Work out the finished part from the listing and answer in its coordinate system (mm). A direction names the side the tool comes from. Coordinates: 2 decimals unless noted, no trailing zeros. Order: outer loops, then holes, each group sorted by start corner. A loop starts at its lowest first (then second) coordinate and runs counter-clockwise, first axis right, second up.
1. The part is cut by section C-C, the plane z = -28. Give the vertices of the cut face in (x, y), then the cut area to 3 significant figures.
2. A tool of negligible diameter and unlimited length cuts with its end or side. For faces 1 (the flat face through (-13.65, 0.02, -21.52)), 2 (the flat face through (-16.895, 0.022, -9.243)), 3 (the flat face through (-14.65, 0.02, -23.84)), 4 (the flat face through (13.61, 0.02, -21.51)), from which of +Z, -Z, +X, -X, +Y, -Y can it reach the whole face along a straight path? Write none if from no direction.
3. The part is cut by section A-A, the plane x = 0. Give the vertices of the cut face in (y, z), then the cut area to 3 significant figures.
4. The part is cut by section D-D, the plane x = -18. Give the vertices of the cut face in (y, z).
5. Find the intervals of material crossed by probe 1 along Z at (x, y) = (0, 0.9); probe 2 along Z at (x, y) = (-2, 1.2); probe 3 along X at (y, z) = (1.1, -21), in increasing order.
6. The part is cut by section B-B, the plane y = -0.05. Give the vertices of the cut face in (x, z), then the cut area to 3 significant figures.
7. Determine the mould class of faces 5 (the flat face through (0, 0, 0)), 6 (the flat face through (19.762, 0.022, -4.762)), 7 (the cylindrical face through (3.53, -0.022, -15.126)), 8 (the flat face through (16.938, 0.022, -9.254)) for opening direction X: +X half, -X half, draft (parallel to the pull), parting line (faces both ways), or undercut.
8. A flat-ended cylindrical pin translates along its axis: pin 1 Ø1 at (y, z) = (0.5, -14.5) entering from -X. Find the tip coordinate at first contact, or state that the pin passes through.
```python
from build123d import *

# Parameters (mm, degrees)
SKETCH1_R           = 7.65
BOSS_EXTRUDE1_DEPTH = 1.5875


with BuildPart() as part:
    # Sketch1 → Boss-Extrude1 (new, symmetric)
    with BuildSketch(Plane(origin=(0, 0, 0), x_dir=(1, 0, 0), z_dir=(0, 1, 0))):
        with BuildLine():
            Line((-18.450042271, 9.659258263), (-21.038232722, 0))
            Line((-21.038232722, 0), (21.038232722, 0))
            Line((21.038232722, 0), (18.450042271, 9.659258263))
            Line((18.450042271, 9.659258263), (15.383227773, 8.837507795))
            Line((15.383227773, 8.837507795), (12.0962259, 21.104765789))
            Line((12.0962259, 21.104765789), (15.163040398, 21.926516257))
            Line((15.163040398, 21.926516257), (14.150813355, 25.704199011))
            ThreePointArc((14.150813355, 25.704199011), (0, 36.5625), (-14.150813355, 25.704199011))
            Line((-14.150813355, 25.704199011), (-15.163040398, 21.926516257))
            Line((-15.163040398, 21.926516257), (-12.0962259, 21.104765789))
            Line((-12.0962259, 21.104765789), (-15.383227773, 8.837507795))
            Line((-15.383227773, 8.837507795), (-18.450042271, 9.659258263))
        make_face()
        with Locations((0, 21.9125)):
            Circle(SKETCH1_R, mode=Mode.SUBTRACT)
    extrude(amount=BOSS_EXTRUDE1_DEPTH, both=True)


solid = part.part
```
Geometry says:
1. outline: (-13.33, -1.59) - (-4.63, -1.59) - (-4.63, 1.59) - (-13.33, 1.59) - close; (4.63, -1.59) - (13.33, -1.59) - (13.33, 1.59) - (4.63, 1.59) - close
1. area: 55.2 mm2
2. face 1: -X, +Y, -Y
2. face 2: -Z, +Y, -Y
2. face 3: -Z, -X, +Y, -Y
2. face 4: +X, +Y, -Y
3. outline: (-1.59, -36.56) - (1.59, -36.56) - (1.59, -29.56) - (-1.59, -29.56) - close; (-1.59, -14.26) - (1.59, -14.26) - (1.59, 0) - (-1.59, 0) - close
3. area: 67.5 mm2
4. outline: (-1.59, -9.54) - (1.59, -9.54) - (1.59, 0) - (-1.59, 0) - close
5. probe 1: z = -36.56 to -29.56, -14.26 to 0
5. probe 2: z = -36.43 to -29.3, -14.53 to 0
5. probe 3: x = -12.12 to -7.6, 7.6 to 12.12
6. outline: (-21.04, 0) - (-18.45, -9.66) - (-15.38, -8.84) - (-12.1, -21.1) - (-15.16, -21.93) - (-14.15, -25.7) arc R14.65 ccw to (14.15, -25.7) - (15.16, -21.93) - (12.1, -21.1) - (15.38, -8.84) - (18.45, -9.66) - (21.04, 0) - close; hole circle Ø15.3 at (0, -21.91)
6. area: 867 mm2
7. face 5: draft
7. face 6: +X half
7. face 7: undercut
7. face 8: undercut
8. pin 1: stops at x = -14
